Source: CAD feature listing. Evaluate the final solid. Frame: model axes, mm. A direction names the side the tool comes from. Round coordinates to 2 decimals unless told otherwise and drop trailing zeros. Loops run counter-clockwise (first coordinate to the right, second up) from the corner with the lowest first, then second, coordinate; pieces in that order, holes last. Notation, with made-up numbers: M -7,-11 L 17,-11 A12 ccw 17,0 Z; hole C -24,72 d5. An arc over 180 degrees is marked long. One line per item, written item: value.
from build123d import *


with BuildPart() as part:
    # Skica1 → Rotovat1 (revolve)
    with BuildSketch(Plane.XY, mode=Mode.PRIVATE) as rotovat1_sk:
        Polygon((8, 64.637455621), (4.5, 64.637455621), (4.5, 52.97460351), (2, 50.637455621), (2, 46.936179321), (2, 31.837455621), (3, 31.837455621), (3, 14.537455621), (12.5, 14.537455621), (12.5, 16.037455621), (7.5, 16.037455621), (7.5, 18.237455621), (12.5, 18.237455621), (12.5, 19.437455621), (7.5, 19.437455621), (7.5, 21.637455621), (12.5, 21.637455621), (12.5, 22.837455621), (7.5, 22.837455621), (7.5, 25.037455621), (12.5, 25.037455621), (12.5, 26.237455621), (7.5, 26.237455621), (7.5, 28.437455621), (12.5, 28.437455621), (12.5, 29.637455621), (7.5, 29.637455621), (7.5, 31.837455621), (12.5, 31.837455621), (12.5, 33.037455621), (6.5, 33.037455621), (6.5, 35.237455621), (12.5, 35.237455621), (12.5, 36.437455621), (4, 36.437455621), (4, 38.637455621), (12.5, 38.637455621), (12.5, 39.837455621), (4, 39.837455621), (4, 42.037455621), (12.5, 42.037455621), (12.5, 43.237455621), (4, 43.237455621), (4, 45.437455621), (12.5, 45.437455621), (12.5, 46.637455621), (4, 46.637455621), (4, 48.837455621), (8, 48.837455621), (8, 50.037455621), (4.5, 50.037455621), (4.5, 51.937455621), (8, 51.937455621), (8, 54.937455621), (6, 54.937455621), (6, 60.937455621), (8, 60.937455621), align=None)
    revolve(rotovat1_sk.sketch.rotate(Axis((0, 64.637455621, 0), (0, -1, 0)), 180), axis=Axis((0, 64.637455621, 0), (0, -1, 0)))


solid = part.part
1. Ray query, line 1 (Z direction, x = 0, y = 62.75); line 2 (Y direction, x = -5.5, z = 2.25); line 3 (Y direction, x = 3.5, z = 2.5). Return the intervals inside material, ascending. Write a range as [from, to].
Report:
line 1: z = [-8, -4.5], [4.5, 8]
line 2: y = [14.54, 36.44], [38.64, 39.84], [42.04, 43.24], [45.44, 46.64], [48.84, 50.04], [51.94, 64.64]
line 3: y = [14.54, 36.44], [38.64, 39.84], [42.04, 43.24], [45.44, 46.64], [48.84, 52.79]
2. Reachability of faces 1 (the face through (3, 46.637, -3)), 2 (the face through (0, 41, 2)), 3 (the face through (1, 31.837, 2)) from +Z, -Z, +X, -X, +Y, -Y: full face, straight path, thin tool, end or side. Return the list, or none.
Report:
face 1: none
face 2: +Y, -Y
face 3: -Y
3. Section query B-B (y = 37). Return the cut outline in (x, z).
Report:
outline: C 0,0 d8; hole C 0,0 d4
4. Pull-direction query (X, two-part tool) for faces 4 (the face through (0, 18.237, 8)), 5 (the face through (3.32, 58.72, -3.04)), 6 (the face through (-4.032, 30.753, -6.324)); classes: released by +X, released by -X, zero draft, split by the parting line, or undercut.
Report:
face 4: zero draft
face 5: undercut
face 6: split by the parting line
5. Pin query (flat end, axial travel): pin 1 (5 mm diameter, centred on x = 4.5, y = 54, fed in from +Z); pin 2 (8 mm diameter, centred on y = 48, z = 6.5, fed in from +X); pin 3 (6 mm diameter, centred on y = 50, z = -3, fed in from -X). Return the tip coordinate at first contact, or that it passes through.
Report:
pin 1: stops at z = 7.75
pin 2: stops at x = 12.2
pin 3: stops at x = -8
6. Section query A-A (x = -10). Count the separate pieces of the cut face and the enclosed holes in it, and give its area (4 significant figures).
Report:
separate pieces: 10
enclosed holes: 0
area: 184.5 mm2
